from build123d import *

# Parameters (mm, degrees)
F1_DEPTH = 6.35
F3_DEPTH = 3.81
F3_TAPER = 3


with BuildPart() as f1:
    # F0 (on Top) → F1 (new body)
    with BuildSketch(Plane.XY):
        with BuildLine():
            Line((12.7, 19.05), (-12.7, 19.05))
            ThreePointArc((-12.7, 19.05), (-17.1901280605, 17.1901280605), (-19.05, 12.7))
            Line((-19.05, 12.7), (-19.05, -12.7))
            ThreePointArc((-19.05, -12.7), (-17.1901280605, -17.1901280605), (-12.7, -19.05))
            Line((-12.7, -19.05), (12.7, -19.05))
            ThreePointArc((12.7, -19.05), (17.1901280605, -17.1901280605), (19.05, -12.7))
            Line((19.05, -12.7), (19.05, 12.7))
            ThreePointArc((19.05, 12.7), (17.1901280605, 17.1901280605), (12.7, 19.05))
        make_face()
    extrude(amount=F1_DEPTH)

    # F2 (on Top) → F3 (join)
    with BuildSketch(Plane.XY):
        with BuildLine():
            ThreePointArc((2.38125, 6.35), (2.1487660076, 6.9112660076), (1.5875, 7.14375))
            Line((1.5875, 7.14375), (-1.5875, 7.14375))
            ThreePointArc((-1.5875, 7.14375), (-2.1487660076, 6.9112660076), (-2.38125, 6.35))
            Line((-2.38125, 6.35), (-2.38125, 2.38125))
            Line((-2.38125, 2.38125), (-6.35, 2.38125))
            ThreePointArc((-6.35, 2.38125), (-6.9112660076, 2.1487660076), (-7.14375, 1.5875))
            Line((-7.14375, 1.5875), (-7.14375, -1.5875))
            ThreePointArc((-7.14375, -1.5875), (-6.9112660076, -2.1487660076), (-6.35, -2.38125))
            Line((-6.35, -2.38125), (-2.38125, -2.38125))
            Line((-2.38125, -2.38125), (-2.38125, -6.35))
            ThreePointArc((-2.38125, -6.35), (-2.1487660076, -6.9112660076), (-1.5875, -7.14375))
            Line((-1.5875, -7.14375), (1.5875, -7.14375))
            ThreePointArc((1.5875, -7.14375), (2.1487660076, -6.9112660076), (2.38125, -6.35))
            Line((2.38125, -6.35), (2.38125, -2.38125))
            Line((2.38125, -2.38125), (6.35, -2.38125))
            ThreePointArc((6.35, -2.38125), (6.9112660076, -2.1487660076), (7.14375, -1.5875))
            Line((7.14375, -1.5875), (7.14375, 1.5875))
            ThreePointArc((7.14375, 1.5875), (6.9112660076, 2.1487660076), (6.35, 2.38125))
            Line((6.35, 2.38125), (2.38125, 2.38125))
            Line((2.38125, 2.38125), (2.38125, 6.35))
        make_face()
        with BuildLine():
            ThreePointArc((5.08, -11.684), (5.0056051224, -11.5043948776), (4.826, -11.43))
            Line((4.826, -11.43), (-4.826, -11.43))
            ThreePointArc((-4.826, -11.43), (-5.0056051224, -11.5043948776), (-5.08, -11.684))
            Line((-5.08, -11.684), (-5.08, -13.716))
            ThreePointArc((-5.08, -13.716), (-5.0056051224, -13.8956051224), (-4.826, -13.97))
            Line((-4.826, -13.97), (4.826, -13.97))
            ThreePointArc((4.826, -13.97), (5.0056051224, -13.8956051224), (5.08, -13.716))
            Line((5.08, -13.716), (5.08, -11.684))
        make_face()
    extrude(amount=-F3_DEPTH, taper=F3_TAPER)


solid = f1.part
The model under review builds one solid part; all positions refer to its coordinate system, in mm. Round coordinates to 2 decimals unless told otherwise and drop trailing zeros. Write each loop counter-clockwise with the first axis right and the second up, starting at its lowest first coordinate (ties: lowest second). Pieces come first, ordered by that corner, then holes. Notation, with made-up numbers: M -33.5,-31.5 L 7.5,-31.5 A19 cw 7.5,-23.5 Z; hole C -8.75,24 d4. An arc over 180 degrees is marked long. Use a Markdown table: item, result. Add a question column.
Q1. To check wall thickness, follow line 1 (Z direction, x = -15.5, y = 4); line 2 (Y direction, x = -3, z = -0.25); line 3 (Y direction, x = 1, z = -0.75). State the ranges of each line that lie inside material, in increasing order.
Q2. We need section A-A, the plane z = 5.75. State the section outline as (x, y) points, plus the area to 3 significant figures.
Q3. We need section B-B, the plane y = 10. State the section outline as (x, z) points, plus the area to 3 significant figures.
Findings below:
| question | item | result |
|---|---|---|
| 1 | line 1 | z = 0 to 6.35 |
| 1 | line 2 | y = -13.96 to -11.44, -2.37 to 2.37 |
| 1 | line 3 | y = -13.93 to -11.47, -7.1 to 7.1 |
| 2 | outline | M -19.05,-12.7 A6.35 ccw -12.7,-19.05 L 12.7,-19.05 A6.35 ccw 19.05,-12.7 L 19.05,12.7 A6.35 ccw 12.7,19.05 L -12.7,19.05 A6.35 ccw -19.05,12.7 Z |
| 2 | area | 1,420 mm² |
| 3 | outline | M -19.05,0 L 19.05,0 L 19.05,6.35 L -19.05,6.35 Z |
| 3 | area | 242 mm² |
